```python
from build123d import *

# Parameters (mm, degrees)
BOSS_EXTRUDE1_DEPTH = 38.1
SKETCH2_R           = 4.52
CUT_EXTRUDE1_DEPTH  = 38.1
SKETCH3_R           = 4.515
CUT_EXTRUDE2_DEPTH  = 10


with BuildPart() as part:
    # Sketch1 → Boss-Extrude1 (new body)
    with BuildSketch(Plane.XY):
        with BuildLine():
            Line((0, 0), (53.98, 0))
            ThreePointArc((53.98, 0), (61.287211447, -2.441393787), (64.401363743, -9.488222735))
            Line((64.401363743, -9.488222735), (64.401363743, -85.721240556))
            ThreePointArc((64.401363743, -85.721240556), (61.664237719, -92.40538322), (55.025128035, -95.25))
            Line((55.025128035, -95.25), (30.071323434, -95.25))
            ThreePointArc((30.071323434, -95.25), (27.161692752, -94.580250085), (24.602099349, -93.043045718))
            Line((24.602099349, -93.043045718), (-7.280670374, -66.290225402))
            Line((-7.280670374, -66.290225402), (-3.198969052, -61.425843189))
            Line((-3.198969052, -61.425843189), (28.68380067, -88.178663504))
            ThreePointArc((28.68380067, -88.178663504), (29.463882201, -88.660646082), (30.349062467, -88.9))
            Line((30.349062467, -88.9), (54.96018039, -88.9))
            ThreePointArc((54.96018039, -88.9), (57.151148485, -87.938216318), (58.051363743, -85.721240556))
            Line((58.051363743, -85.721240556), (58.051363743, -9.488222735))
            ThreePointArc((58.051363743, -9.488222735), (56.930321756, -7.064776449), (54.357595252, -6.35))
            Line((54.357595252, -6.35), (0, -6.35))
            Line((0, -6.35), (0, 0))
        make_face()
    extrude(amount=BOSS_EXTRUDE1_DEPTH)

    # Sketch2 → Cut-Extrude1 (cut)
    with BuildSketch(Plane(origin=(0, 0, 0), x_dir=(1, 0, 0), z_dir=(0, 1, 0))):
        with Locations((24.5, -19.05)):
            Circle(SKETCH2_R)
    extrude(amount=-CUT_EXTRUDE1_DEPTH, mode=Mode.SUBTRACT)

    # Sketch3 → Cut-Extrude2 (cut)
    with BuildSketch(Plane(origin=(-35.649761578, -42.485731436, 0), x_dir=(0.766044443, -0.64278761, 0), z_dir=(-0.64278761, -0.766044443, 0))):
        with Locations((57.84321845, 19.05)):
            Circle(SKETCH3_R)
    extrude(amount=-CUT_EXTRUDE2_DEPTH, mode=Mode.SUBTRACT)


solid = part.part
```
Could you check a few things on this model? Use its own coordinates, in mm. A direction names the side the tool comes from. Give positions to 0.01 mm unless a question says otherwise; leave off trailing zeros. Order: outer loops, then holes, each group sorted by start corner. A loop starts at its lowest first (then second) coordinate and runs counter-clockwise, first axis right, second up.
Q1. For faces 1 (the flat face through (61, -47, 38.1)), 2 (the flat face through (58.051, -48, 19)), 3 (the flat face through (0, -3, 19)), 4 (the flat face through (28, -6.35, 23)), 5 (the cylindrical face through (19.984, -3.131, 18.851)), which set-ups out of +Z, -Z, +X, -X, +Y, -Y let a thin tool reach every point of the face, with its end or its side?
Q2. Suppose I cut it at A-A, the plane x = 41. Write out the boundary of the cut face in (y, z).
Q3. I'm going to push flat-ended pins straight in: P1, Ø10.5, axis at x = 24.5, z = 19.05, coming from the -Y side; P2, Ø5, axis at y = -2.5, z = 12.5, coming from the -X side; P3, Ø19, axis at x = 32, z = 17, coming from the +Y side. Where does each tip first touch, or does it pass through?
Q4. Suppose I cut it at C-C, the plane y = -63.5. Write out the boundary of the cut face in (x, z).
Q5. Suppose I cut it at D-D, the plane z = 3. Write out the boundary of the cut face in (x, y).
Q6. We'd pull the mould along X, two halves only. Please class faces 6 (the flat face through (64.401, -47, 19)), 7 (the cylindrical face through (57.13, -87.96, 18.78)), 8 (the flat face through (12.43, -82.83, 18.78)): +X half, -X half, draft (parallel to the pull), parting line (faces both ways), or undercut.
Q7. Suppose I cut it at B-B, the plane z = 18. Write out the boundary of the cut face in (x, y), and give its area (3 significant figures).
Q8. If I drill on line 1 along Y through (x, z) = (38, 36.5); line 2 along Z through (x, y) = (24, -2), over which ranges is the centre line in solid material (lowest first)?
Solution:
1. face 1: +Z, +X, -X, +Y, -Y
1. face 2: +Z, -Z
1. face 3: +Z, -Z, -X, +Y
1. face 4: +Z, -Z, -X
1. face 5: +Y
2. outline: (-95.25, 0) - (-88.9, 0) - (-88.9, 38.1) - (-95.25, 38.1) - close; (-6.35, 0) - (0, 0) - (0, 38.1) - (-6.35, 38.1) - close
3. P1: stops at y = -95.22
3. P2: stops at x = 0
3. P3: stops at y = 0
4. outline: (-4.94, 0) - (-0.73, 0) - (-0.73, 38.1) - (-4.94, 38.1) - close; (58.05, 0) - (64.4, 0) - (64.4, 38.1) - (58.05, 38.1) - close
5. outline: (-7.28, -66.29) - (24.6, -93.04) arc R9.53 ccw to (30.07, -95.25) - (55.03, -95.25) arc R9.53 ccw to (64.4, -85.72) - (64.4, -9.49) arc R9.53 ccw to (53.98, 0) - (0, 0) - (0, -6.35) - (54.36, -6.35) arc R3.18 cw to (58.05, -9.49) - (58.05, -85.72) arc R3.18 cw to (54.96, -88.9) - (30.35, -88.9) arc R3.18 cw to (28.68, -88.18) - (-3.2, -61.43) - close
6. face 6: +X half
6. face 7: undercut
6. face 8: -X half
7. outline: (-7.28, -66.29) - (5.3, -76.84) - (9.38, -71.98) - (-3.2, -61.43) - close; (0, -6.35) - (20.1, -6.35) - (20.1, 0) - (0, 0) - close; (12.02, -82.49) - (24.6, -93.04) arc R9.53 ccw to (30.07, -95.25) - (55.03, -95.25) arc R9.53 ccw to (64.4, -85.72) - (64.4, -9.49) arc R9.53 ccw to (53.98, 0) - (28.9, 0) - (28.9, -6.35) - (54.36, -6.35) arc R3.18 cw to (58.05, -9.49) - (58.05, -85.72) arc R3.18 cw to (54.96, -88.9) - (30.35, -88.9) arc R3.18 cw to (28.68, -88.18) - (16.11, -77.62) - close
7. area: 1,290 mm2
8. line 1: y = -95.25 to -88.9, -6.35 to 0
8. line 2: z = 0 to 14.56, 23.54 to 38.1
